For this review, take the finished solid that the model builds, in its own axes (mm). A direction names the side the tool comes from. Give positions to 0.01 mm unless a question says otherwise; leave off trailing zeros. Order: outer loops, then holes, each group sorted by start corner. A loop starts at its lowest first (then second) coordinate and runs counter-clockwise, first axis right, second up. Notation, with made-up numbers: (-14, 55.25) - (7, 55.25) arc R12 ccw to (7, 78.25) - close; hole circle Ø1 at (79, 80.25). An arc over 180 degrees is marked (long way). One line per item, written item: value.
```python
from build123d import *
from build123d.topology import SkipClean

# Parameters (mm, degrees)
SKETCH1_R           = 11.873640169
BOSS_EXTRUDE1_DEPTH = 25.4
BOSS_EXTRUDE2_DEPTH = 4.359372013
SKETCH3_W           = 23.747280338
SKETCH3_H           = 63.5
BOSS_EXTRUDE3_DEPTH = 20.377197654
SKETCH6_W           = 23.747280338
SKETCH6_H           = 58.477197654
BOSS_EXTRUDE4_DEPTH = 2.179686006
SKETCH7_W           = 23.747280338
SKETCH7_H           = 58.477197654
BOSS_EXTRUDE5_DEPTH = 2.179686006
SKETCH8_W           = 23.747280338
SKETCH8_H           = 27.579686006
BOSS_EXTRUDE6_DEPTH = 18.991849144


with BuildPart() as part:
    # Sketch1 → Boss-Extrude1 (new body)
    with BuildSketch(Plane.YZ):
        with Locations(Location((0, 0, 0), (0, 0, 270))):
            Circle(SKETCH1_R)
    extrude(amount=BOSS_EXTRUDE1_DEPTH)

    # Sketch2 → Boss-Extrude2 (add)
    with SkipClean():  # the faces are left unmerged after this step: merging them gives an invalid solid
        with BuildSketch(Plane.YZ.offset(25.4)):
            with BuildLine():
                Line((-11.873640169, -1.316e-06), (-11.873640169, 38.099998684))
                Line((-11.873640169, 38.099998684), (11.873640169, 38.099998684))
                Line((11.873640169, 38.099998684), (11.873640169, 0))
                ThreePointArc((11.873640169, 0), (6.58e-07, -11.873640169), (-11.873640169, -1.316e-06))
            make_face()
        extrude(amount=BOSS_EXTRUDE2_DEPTH)
    add(part.part.scale(1), mode=Mode.REPLACE)  # the faces are merged on a copy

    # Sketch3 → Boss-Extrude3 (add)
    with BuildSketch(Plane.XY.offset(38.099998684)):
        with Locations((17.885731844, 0)):
            Rectangle(SKETCH3_W, SKETCH3_H)
    extrude(amount=BOSS_EXTRUDE3_DEPTH)

    # Sketch6 → Boss-Extrude4 (add)
    with BuildSketch(Plane(origin=(0, 31.75, 0), x_dir=(-1, 0, 0), z_dir=(0, 1, 0))):
        with Locations((-17.885731844, 67.338597511)):
            Rectangle(SKETCH6_W, SKETCH6_H)
    extrude(amount=BOSS_EXTRUDE4_DEPTH)

    # Sketch7 → Boss-Extrude5 (add)
    with BuildSketch(Plane.XZ.offset(31.75)):
        with Locations((17.885731844, 67.338597511)):
            Rectangle(SKETCH7_W, SKETCH7_H)
    extrude(amount=BOSS_EXTRUDE5_DEPTH)

    # Sketch8 → Boss-Extrude6 (add)
    with BuildSketch(Plane.XY.offset(96.577196338)):
        with Locations((17.885731844, 20.139843003)):
            Rectangle(SKETCH8_W, SKETCH8_H)
        with Locations((17.885731844, -20.139843003)):
            Rectangle(SKETCH8_W, SKETCH8_H)
    extrude(amount=BOSS_EXTRUDE6_DEPTH)


solid = part.part
```
(1) Take a section at C-C (z = 95). Write out the cut boundary in (x, y).
Answers below:
outline: (6.01, -33.93) - (29.76, -33.93) - (29.76, -31.75) - (6.01, -31.75) - close; (6.01, 31.75) - (29.76, 31.75) - (29.76, 33.93) - (6.01, 33.93) - close
(2) Take a section at A-A (x = 13.25). Write out the cut boundary in (y, z), then the cut area to 3 significant figures.
Answers below:
outline: (-33.93, 38.1) - (33.93, 38.1) - (33.93, 115.57) - (6.35, 115.57) - (6.35, 96.58) - (31.75, 96.58) - (31.75, 58.48) - (-31.75, 58.48) - (-31.75, 96.58) - (-6.35, 96.58) - (-6.35, 115.57) - (-33.93, 115.57) - close; circle Ø23.75 at (0, 0)
area: 3,040 mm^2
(3) Draft analysis for pull direction Y (two halves, no side actions). For faces 1 (the face through (28, 11.874, 19)), 2 (the face through (25.4, 0, 24)), 3 (the face through (18, -31.75, 78)), state which applies: pulls with the +Y half, pulls with the -Y half, needs draft (parallel to the pull), parting line crosses it, or undercut.
Answers below:
face 1: pulls with the +Y half
face 2: needs draft
face 3: undercut
(4) Take a section at B-B (y = 21). Write out the cut boundary in (x, z).
Answers below:
outline: (6.01, 38.1) - (29.76, 38.1) - (29.76, 58.48) - (6.01, 58.48) - close; (6.01, 96.58) - (29.76, 96.58) - (29.76, 115.57) - (6.01, 115.57) - close
(5) Machinability: for faces 4 (the face through (6.012, 0, 50)), 5 (the face through (18, 33.93, 76)), 6 (the face through (28, -11.874, 19)), 7 (the face through (18, 6.35, 106)), 8 (the face through (18, 31.75, 78)), which of the approach directions +Z, -Z, +X, -X, +Y, -Y give a long, thin tool a straight path to every point of the face, cutting with its end or side? Answer none if there is none.
Answers below:
face 4: +Z, -X, +Y, -Y
face 5: +Z, -Z, +X, -X, +Y
face 6: -Z, +X, -X, -Y
face 7: +Z, +X, -X
face 8: +X, -X
(6) For P1, Ø8, axis at x = 18.5, z = 5.5, coming from the -Y side; P2, Ø3, axis at x = 24.5, y = 21.5, coming from the -Z side; P3, Ø1.3, axis at x = 27, z = 19.5, coming from the +Y side, all flat-tipped, find the tip position at first contact; note any pin that passes through.
Answers below:
P1: stops at y = -11.78
P2: stops at z = 38.1
P3: stops at y = 11.87
(7) Take a section at D-D (y = 0). Write out the cut boundary in (x, z).
Answers below:
outline: (0, -11.87) - (29.76, -11.87) - (29.76, 58.48) - (6.01, 58.48) - (6.01, 38.1) - (25.4, 38.1) - (25.4, 11.87) - (0, 11.87) - close
(8) Wall thickness on line 1 (Z direction, x = 14, y = -21); line 2 (Y direction, x = 8.25, z = 81); line 3 (Y direction, x = 27, z = 9): over which ranges is each line inside the solid? List them lowest first. Write a range as from..to.
Answers below:
line 1: z = 38.1..58.48, 96.58..115.57
line 2: y = -33.93..-31.75, 31.75..33.93
line 3: y = -11.87..11.87
